Input: part model. Units: mm. Frame: model coordinates. Face numbers are marked on the shaded views. A direction names the side the tool comes from. Give positions to 0.01 mm unless a question says otherwise; leave off trailing zeros. Order: outer loops, then holes, each group sorted by start corner. A loop starts at its lowest first (then second) coordinate and runs counter-clockwise, first axis right, second up.
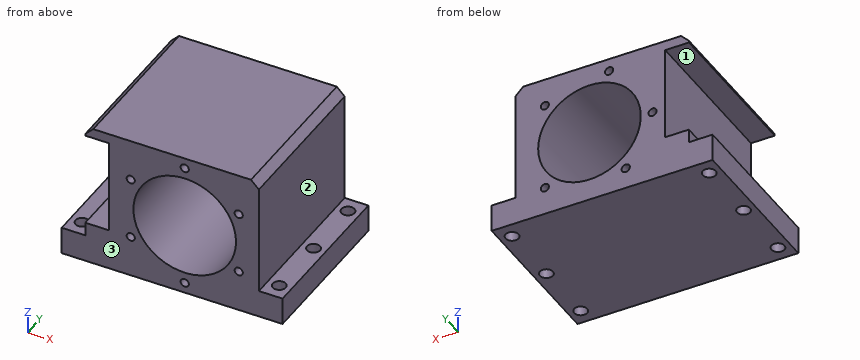
```python
from build123d import *

# Parameters (mm, degrees)
SKETCH_1_W           = 140
SKETCH_1_H           = 100
EXTRUDE_1_DEPTH      = 92.5
SKETCH_2_R           = 32.525
CUT_EXTRUDE_1_DEPTH  = 101
SKETCH_3_OUTSIDE_W   = 181.068
SKETCH_3_OUTSIDE_H   = 141.068
SKETCH_3_OUTSIDE_W_2 = 110
SKETCH_3_OUTSIDE_H_2 = 100
CUT_EXTRUDE_2_DEPTH  = 75
SKETCH_5_W           = 60.05
SKETCH_5_H           = 100
CUT_EXTRUDE_3_DEPTH  = 15
CHAMFER_2_SIZE       = 5
SKETCH_6_R           = 2.6
CUT_EXTRUDE_4_DEPTH  = 20
SKETCH_9_R           = 4.15
CUT_EXTRUDE_5_DEPTH  = 18.5
SKETCH_10_R          = 2.6
CUT_EXTRUDE_6_DEPTH  = 20


with BuildPart() as part:
    # 草图1 → 凸台-拉伸1 (new body)
    with BuildSketch(Plane.XY):
        with Locations((70, -50)):
            Rectangle(SKETCH_1_W, SKETCH_1_H)
    extrude(amount=EXTRUDE_1_DEPTH)

    # 草图2 → 切除-拉伸1 (cut, through all)
    with BuildSketch(Plane(origin=(0, 0, 0), x_dir=(1, 0, 0), z_dir=(0, 1, 0))):
        with Locations((78, -46.25)):
            Circle(SKETCH_2_R)
    extrude(amount=-CUT_EXTRUDE_1_DEPTH, mode=Mode.SUBTRACT)

    # 草图3 outside → 切除-拉伸2 (cut)
    with BuildSketch(Plane.XY.offset(92.5)):
        with Locations((70, -50)):
            Rectangle(SKETCH_3_OUTSIDE_W, SKETCH_3_OUTSIDE_H)
        with Locations((70, -50)):
            Rectangle(SKETCH_3_OUTSIDE_W_2, SKETCH_3_OUTSIDE_H_2, mode=Mode.SUBTRACT)
    extrude(amount=-CUT_EXTRUDE_2_DEPTH, mode=Mode.SUBTRACT)

    # 草图5 → 切除-拉伸3 (cut)
    with BuildSketch(Plane.ZY.offset(-15)):
        with Locations((56.225, -50)):
            Rectangle(SKETCH_5_W, SKETCH_5_H)
    extrude(amount=-CUT_EXTRUDE_3_DEPTH, mode=Mode.SUBTRACT)

    # 倒角2
    chamfer_2_edges = [part.edges().sort_by_distance(p)[0] for p in [
        (15, -50, 92.5),
        (125, -50, 92.5),
    ]]
    chamfer(chamfer_2_edges, length=CHAMFER_2_SIZE)

    # 草图6 → 切除-拉伸4 (cut)
    with BuildSketch(Plane.XZ.offset(100)):
        with Locations((78, 85.75)):
            Circle(SKETCH_6_R)
        with Locations((112.208003449, 66)):
            Circle(SKETCH_6_R)
        with Locations((112.208003449, 26.5)):
            Circle(SKETCH_6_R)
        with Locations((78, 6.75)):
            Circle(SKETCH_6_R)
        with Locations((43.791996551, 26.5)):
            Circle(SKETCH_6_R)
        with Locations((43.791996551, 66)):
            Circle(SKETCH_6_R)
    extrude(amount=-CUT_EXTRUDE_4_DEPTH, mode=Mode.SUBTRACT)

    # 草图9 → 切除-拉伸5 (cut, through all)
    with BuildSketch(Plane.XY.offset(17.5)):
        with Locations((7.5, -10)):
            Circle(SKETCH_9_R)
        with Locations((132.5, -10)):
            Circle(SKETCH_9_R)
        with Locations((132.5, -50)):
            Circle(SKETCH_9_R)
        with Locations((132.5, -90)):
            Circle(SKETCH_9_R)
        with Locations((7.5, -50)):
            Circle(SKETCH_9_R)
        with Locations((7.5, -90)):
            Circle(SKETCH_9_R)
    extrude(amount=-CUT_EXTRUDE_5_DEPTH, mode=Mode.SUBTRACT)

    # 草图10 → 切除-拉伸6 (cut)
    with BuildSketch(Plane(origin=(0, 0, 0), x_dir=(1, 0, 0), z_dir=(0, 1, 0))):
        with Locations((106.284271247, -17.965728753)):
            Circle(SKETCH_10_R)
        with Locations((106.284271247, -74.534271247)):
            Circle(SKETCH_10_R)
        with Locations((38, -46.25)):
            Circle(SKETCH_10_R)
        with Locations((65.534490363, -84.258039538)):
            Circle(SKETCH_10_R)
        with Locations((55.025808003, -13.505740929)):
            Circle(SKETCH_10_R)
    extrude(amount=-CUT_EXTRUDE_6_DEPTH, mode=Mode.SUBTRACT)


solid = part.part
```
1) Cut plane B-B (x = 78). Return the cut outline in (y, z) (3 decimals), then the cut area to 3 significant figures.
2) Line query: probe 1 along X at (y, z) = (-89.5, 65); probe 2 along Z at (x, y) = (24, -55); probe 3 along X at (y, z) = (-86.5, 42). Output: solid intervals per line, ascending.
3) Cut plane A-A (y = -50). Return the cut outline in (x, z) (3 decimals).
4) Cut plane D-D (z = 6.75). Return the cut outline in (x, y).
5) First-contact query: P1, Ø2.5, axis at x = 78, z = 84.5, coming from the -Y side; P2, Ø12, axis at x = 51, z = 25, coming from the +Y side; P3, Ø2.5, axis at x = 38, z = 45.5, coming from the +Y side; P4, Ø8, axis at y = -55.5, z = 74.5, coming from the -X side. Flat tips, straight axial feed; report the tip coordinate or a pass-through.
6) Reachability of the marked faces 1, 2 and 3 from +Z, -Z, +X, -X, +Y, -Y: full face, straight path, thin tool, end or side. Return the list, or none.
7) Cut plane C-C (y = -90). Count the separate pieces of the cut face and the enclosed holes in it, then the cut area to 3 significant figures.
Geometry says:
1. outline: (-100, 0) - (0, 0) - (0, 13.725) - (-100, 13.725) - (-100, 9.35) - (-80, 9.35) - (-80, 4.15) - (-100, 4.15) - close; (-100, 78.775) - (0, 78.775) - (0, 92.5) - (-100, 92.5) - (-100, 88.35) - (-80, 88.35) - (-80, 83.15) - (-100, 83.15) - close
1. area: 2,540 mm2
2. probe 1: x = 30 to 41.39, 46.19 to 51.42, 104.58 to 109.81, 114.61 to 125
2. probe 2: z = 0 to 26.2, 86.25 to 92.5
2. probe 3: x = 30 to 45.75, 110.25 to 125
3. outline: (0, 0) - (3.35, 0) - (3.35, 17.5) - (0, 17.5) - close; (11.65, 0) - (128.35, 0) - (128.35, 17.5) - (125, 17.5) - (125, 87.5) - (120, 92.5) - (20, 92.5) - (15, 87.5) - (15, 86.25) - (30, 86.25) - (30, 26.2) - (15, 26.2) - (15, 17.5) - (11.65, 17.5) - close; (136.65, 0) - (140, 0) - (140, 17.5) - (136.65, 17.5) - close; hole circle Ø65.05 at (78, 46.25)
4. outline: (0, -100) - (75.4, -100) - (75.4, -80) - (80.6, -80) - (80.6, -100) - (140, -100) - (140, 0) - (0, 0) - close; hole circle Ø8.3 at (7.5, -90); hole circle Ø8.3 at (7.5, -50); hole circle Ø8.3 at (7.5, -10); hole circle Ø8.3 at (132.5, -90); hole circle Ø8.3 at (132.5, -50); hole circle Ø8.3 at (132.5, -10)
5. P1: stops at y = -80
5. P2: stops at y = 0
5. P3: stops at y = -20
5. P4: stops at x = 30
6. face 1: -X, +Y, -Y
6. face 2: +Z, +X, +Y, -Y
6. face 3: +Z, -Z, +X, -X, -Y
7. separate pieces: 3
7. enclosed holes: 7
7. area: 6,030 mm2
